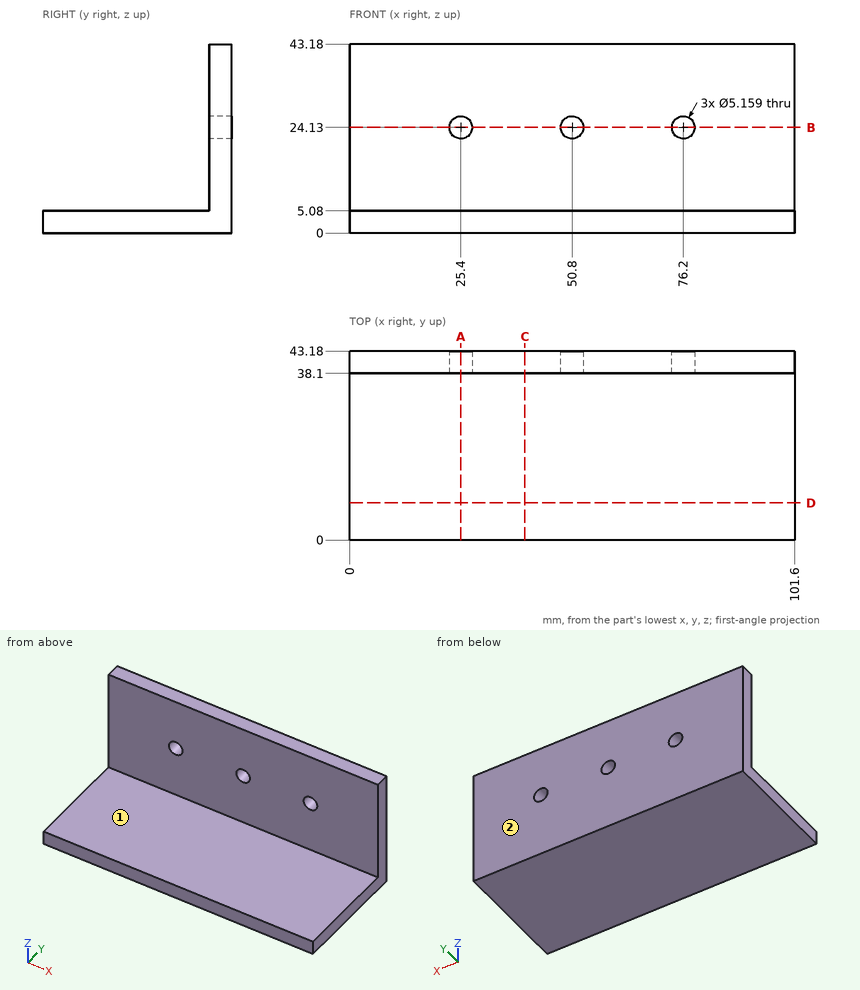
Input: dimensioned drawing with shaded views. Units: mm. Origin: part minimum x, y, z. A direction names the side the tool comes from. Give positions to 0.01 mm unless a question says otherwise; leave off trailing zeros. Write each loop counter-clockwise with the first axis right and the second up, starting at its lowest first coordinate (ties: lowest second). Pieces come first, ordered by that corner, then holes. Notation, with made-up numbers: (72.5, 78) -> (126.5, 78) arc R23 ccw to (126.5, 108) -> close; hole circle Ø8 at (46, 16.25). An arc over 180 degrees is marked (long way). Return JSON: item names as keys, results as strings. Group by question number.
1. Material intervals for line 1 (X direction, y = 41, z = 24); line 2 (Z direction, x = 50.8, y = 39.45); line 3 (Z direction, x = 77.5, y = 7.5), sorted ascending. Write a range as from..to.
2. Section B-B, the plane z = 24.13. Output: boundary loops of the cut face in (x, y).
3. Section A-A, the plane x = 25.4. Output: boundary loops of the cut face in (y, z).
4. Section D-D, the plane y = 8.5. Output: boundary loops of the cut face in (x, z), then the cut area to 3 significant figures.
5. Pin query (flat end, axial travel): pin 1 Ø8 at (x, y) = (83.5, 6) entering from +Z; pin 2 Ø19 at (x, z) = (49, 24) entering from -Y. Return the tip coordinate at first contact, or that it passes through.
6. Section C-C, the plane x = 40. Output: boundary loops of the cut face in (y, z), then the cut area to 3 significant figures.
7. Access query for the marked faces 1 and 2. Directions: +Z, -Z, +X, -X, +Y, -Y. A direction counts if a zero-diameter tool reaches every point of the face in a straight line with its end or side. Return the directions, or none.
Determined:
{
 "1": {"line 1": "x = 0..22.82, 27.98..48.22, 53.38..73.62, 78.78..101.6", "line 2": "z = 0..21.55, 26.71..43.18", "line 3": "z = 0..5.08"},
 "2": {"outline": "(0, 38.1) -> (22.82, 38.1) -> (22.82, 43.18) -> (0, 43.18) -> close; (27.98, 38.1) -> (48.22, 38.1) -> (48.22, 43.18) -> (27.98, 43.18) -> close; (53.38, 38.1) -> (73.62, 38.1) -> (73.62, 43.18) -> (53.38, 43.18) -> close; (78.78, 38.1) -> (101.6, 38.1) -> (101.6, 43.18) -> (78.78, 43.18) -> close"},
 "3": {"outline": "(0, 0) -> (43.18, 0) -> (43.18, 21.55) -> (38.1, 21.55) -> (38.1, 5.08) -> (0, 5.08) -> close; (38.1, 26.71) -> (43.18, 26.71) -> (43.18, 43.18) -> (38.1, 43.18) -> close"},
 "4": {"outline": "(0, 0) -> (101.6, 0) -> (101.6, 5.08) -> (0, 5.08) -> close", "area": "516 mm2"},
 "5": {"pin 1": "stops at z = 5.08", "pin 2": "stops at y = 38.1"},
 "6": {"outline": "(0, 0) -> (43.18, 0) -> (43.18, 43.18) -> (38.1, 43.18) -> (38.1, 5.08) -> (0, 5.08) -> close", "area": "413 mm2"},
 "7": {"face 1": "+Z, +X, -X, -Y", "face 2": "+Z, -Z, +X, -X, +Y"}
}
